For this review, take the finished solid that the model builds, in its own axes (mm). Round coordinates to 2 decimals unless told otherwise and drop trailing zeros. Write each loop counter-clockwise with the first axis right and the second up, starting at its lowest first coordinate (ties: lowest second). Pieces come first, ordered by that corner, then holes. Notation, with made-up numbers: (-29, 76) -> (25, 76) arc R15 cw to (25, 96) -> close; hole circle Ø11 at (22.5, 42). An arc over 180 degrees is marked (long way). Answer in a Markdown table with one row per item.
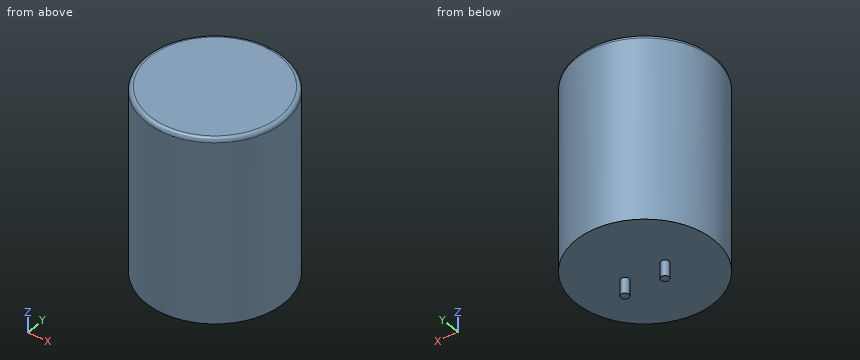
Autodesk Inventor part; units mm, degrees
ref_plane "Arbeitsebene1" through (0, 0, 0) normal (0, 1, 0) x (-1, 0, 0)
ref_plane "YZ Plane" through (0, 0, 0) normal (1, 0, 0) x (0, 1, 0)
ref_plane "XY Plane" through (0, 0, 0) normal (0, 0, 1) x (1, 0, 0)
sketch "Skizze1" plane through (0, 0, 0) normal (0, 0, 1) x (1, 0, 0)
  circle A0 centre (0, 0) radius 17.5
  dimension "d0" = 35
extrude "Extrusion1" add sketch "Skizze1" along normal blind 47
fillet "Rundung1" radius 1 1 edges at (-17.5, 0, 47)
sketch "Skizze2" plane through (0, 0, 0) normal (0, 0, -1) x (-1, 0, 0)
  line L0 (-24.5, 0) -> (24.5, 0)
  line L1 (0, -24.5) -> (0, 24.5)
  circle A0 centre (-5, 0) radius 1
  circle A1 centre (5, 0) radius 1
  dimension "d4" = 10
  dimension "d5" = 2
extrude "Extrusion2" add sketch "Skizze2" along normal blind 4
ref_plane "Arbeitsebene1" through (0, 0, 0) normal (0, 1, 0) x (-1, 0, 0)
properties part number "Kondensator 30x50" material "PC/ABS-Kunststoff"
1) For line 1 (Z direction, x = -14, y = -8); line 2 (X direction, y = -0.5, z = 27); line 3 (X direction, y = -1.5, z = 31), list the stretches that pass through material, from the lowest coordinate up. Write a range as [from, to].
Solved:
| item | result |
|---|---|
| line 1 | [0, 47] |
| line 2 | [-17.49, 17.49] |
| line 3 | [-17.44, 17.44] |
2) Consider section A-A on y = 0. State the section outline as (x, z) points, then the cut area to 3 significant figures.
Solved:
| item | result |
|---|---|
| outline | (-17.5, 0) -> (-6, 0) -> (-6, -4) -> (-4, -4) -> (-4, 0) -> (4, 0) -> (4, -4) -> (6, -4) -> (6, 0) -> (17.5, 0) -> (17.5, 46) arc R1 ccw to (16.5, 47) -> (-16.5, 47) arc R1 ccw to (-17.5, 46) -> close |
| area | 1,660 mm² |
3) Consider section C-C on z = 30.5. State the section outline as (x, y) points, then the cut area to 3 significant figures.
Solved:
| item | result |
|---|---|
| outline | circle Ø35 at (0, 0) |
| area | 962 mm² |
4) Consider section B-B on x = 0. State the section outline as (y, z) points.
Solved:
| item | result |
|---|---|
| outline | (-17.5, 0) -> (17.5, 0) -> (17.5, 46) arc R1 ccw to (16.5, 47) -> (-16.5, 47) arc R1 ccw to (-17.5, 46) -> close |
5) Clearance check with flat-ended pins moving along their axes: pin 1 Ø3 at (y, z) = (-8, 5) entering from +X; pin 2 Ø5 at (x, z) = (-9, 25.5) entering from +Y; pin 3 Ø8 at (x, z) = (-1.5, 25) entering from -Y; pin 4 Ø4 at (y, z) = (8.5, 1.5) entering from -X. State where each tip first meets the part, or that it passes through.
Solved:
| item | result |
|---|---|
| pin 1 | x = 16.25 |
| pin 2 | y = 16.25 |
| pin 3 | y = -17.5 |
| pin 4 | x = -16.25 |
